Autodesk Inventor part; units mm, degrees
ref_plane "Work Plane1" through (1.7107, 0, 1.8263) normal (1, 0, 0) x (0, 0, -1)
ref_plane "YZ Plane" through (0, 0, 0) normal (1, 0, 0) x (0, 1, 0)
ref_plane "XZ Plane" through (0, 0, 0) normal (0, 1, 0) x (-1, 0, 0)
sketch "Sketch1" plane through (0, 0, 0) normal (0, 1, 0) x (-1, 0, 0)
  line L0 (0, 0) -> (2.6987, 0) construction
  line L1 (2.6987, 0) -> (2.6987, -2.7407) construction
  line L2 (2.6987, -2.7407) -> (0, -2.7407) construction
  line L3 (0, -2.7407) -> (0, 0) construction
  line L4 (2.6987, 0) -> (2.6987, -1.8263) construction
  line L5 (2.6987, 0) -> (4.525, 0) construction
  arc A0 (0, -2.7407) -> (2.6987, -1.8263) centre (0, 1.6991) ccw
  line L6 (2.6987, -1.8263) -> (2.6987, 0)
  arc A1 (-2.6987, -1.8263) -> (0, -2.7407) centre (0, 1.6991) ccw
  line L7 (-2.6987, -1.8263) -> (-2.6987, 0)
  arc A2 (2.6987, 1.8263) -> (0, 2.7407) centre (0, -1.6991) ccw
  line L8 (2.6987, 1.8263) -> (2.6987, 0)
  arc A3 (0, 2.7407) -> (-2.6987, 1.8263) centre (0, -1.6991) ccw
  line L9 (-2.6987, 1.8263) -> (-2.6987, 0)
  dimension "d0" = 2.6987
  dimension "d1" = 2.7407
  dimension "d2" = 1.8263
  dimension "d3" = 90
extrude "Extrusion1" add sketch "Sketch1" along normal blind 7.8334
sketch "Sketch2" plane through (0, 0, 0) normal (0, -1, 0) x (1, 0, 0)
  circle A0 centre (0, 0) radius 1.5862
  dimension "d6" = 3.1725
extrude "Extrusion2" cut sketch "Sketch2" against normal blind 4.0589
ref_plane "Work Plane1" through (1.7107, 0, 1.8263) normal (1, 0, 0) x (0, 0, -1)
sketch "Sketch3" plane through (1.7107, 0, 1.8263) normal (1, 0, 0) x (0, 0, -1)
  line L0 (3.6525, 7.8334) -> (0, 7.8334)
  line L1 (3.6525, 7.8334) -> (0, 7.8334)
  line L2 (0, 7.8334) -> (0, 9.3066)
  line L3 (0, 9.3066) -> (1.8263, 9.3066) construction
  line L4 (3.6525, 9.3066) -> (3.6525, 7.8334)
  arc A0 (0.7459, 12.8145) -> (2.9066, 12.8145) centre (1.8263, 11.7342) ccw
  line L5 (1.8263, 11.7342) -> (1.8263, 14.772) construction
  line L6 (2.9066, 12.8145) -> (3.9743, 13.8822)
  line L7 (0.7459, 12.8145) -> (-0.3218, 13.8822)
  arc A1 (-0.3218, 13.8822) -> (0, 9.3066) centre (1.8263, 11.7342) ccw
  arc A2 (3.6525, 9.3066) -> (3.9743, 13.8822) centre (1.8263, 11.7342) ccw
  point P0 (1.8263, 0)
  dimension "d10" = 1.4732
  dimension "d12" = 3.0556
  dimension "d13" = 45
  dimension "d14" = 45
extrude "Extrusion3" add sketch "Sketch3" against normal blind 3.2385
properties part number "hand project" material "ABS Plastic"
The model under review builds one solid part; all positions refer to its coordinate system, in mm. A direction names the side the tool comes from. Give positions to 0.01 mm unless a question says otherwise; leave off trailing zeros. Write each loop counter-clockwise with the first axis right and the second up, starting at its lowest first coordinate (ties: lowest second). Pieces come first, ordered by that corner, then holes.
(1) Consider section A-A, the plane y = 2.75. Give the boundary of the cut face in (x, z).
(2) For P1, Ø1.2, axis at x = -0.5, y = 8.5, coming from the +Z side; P2, Ø2.5, axis at x = 0.5, z = 0.5, coming from the +Y side; P3, Ø0.7, axis at x = 0.5, y = 8.5, coming from the -Z side; P4, Ø3, axis at x = 2, z = 1.5, coming from the -Y side, all flat-tipped, find the tip position at first contact; note any pin that passes through.
(3) To check wall thickness, follow L1, parallel to Z at x = 0, y = 1.25; L2, parallel to Y at x = -2.1, z = 0; L3, parallel to X at y = 10.5, z = -1.75. State the ranges of each line that lie inside material, in increasing order.
(4) The part is to be moulded in two halves that separate along Z. For faces 5 (the cylindrical face through (0.114, 10.207, 0.05)), 6 (the flat face through (0, 9, 1.826)), 7 (the flat face through (-1.528, 10, -1)), say which applies: released by +Z, released by -Z, zero draft, split by the parting line, or undercut.
(5) Consider section B-B, the plane z = -2.5. Give the boundary of the cut face in (x, y), and give its area (3 significant figures).
(6) Tool access review of faces 1 (the cylindrical face through (-1.44, 3.86, -2.5)), 2 (the cylindrical face through (1.41, 3.86, -2.51)), 3 (the flat face through (0, 9, -1.826)), 4 (the cylindrical face through (-0.34, 2, -1.55)): name each direction out of +Z, -Z, +X, -X, +Y, -Y from which nothing blocks a thin tool from reaching the whole face with its end or side.
(7) Consider section D-D, the plane z = 0. Give the boundary of the cut face in (x, y), and give its area (3 significant figures).
(8) Consider section C-C, the plane y = 11.5. Give the boundary of the cut face in (x, z), and give its area (3 significant figures).
Returned:
1. outline: (-2.7, -1.83) arc R4.44 ccw to (0, -2.74) arc R4.44 ccw to (2.7, -1.83) - (2.7, 1.83) arc R4.44 ccw to (0, 2.74) arc R4.44 ccw to (-2.7, 1.83) - close; hole circle Ø3.17 at (0, 0)
2. P1: stops at z = 1.83
2. P2: stops at y = 13.48
2. P3: stops at z = -1.83
2. P4: stops at y = 0
3. L1: z = -2.74 to -1.59, 1.59 to 2.74
3. L2: y = 0 to 7.83
3. L3: x = -1.53 to 1.71
4. face 5: undercut
4. face 6: released by +Z
4. face 7: zero draft
5. outline: (-1.53, 10.01) - (1.71, 10.01) - (1.71, 13.46) - (-1.53, 13.46) - close; (-1.44, 0) - (1.44, 0) - (1.44, 7.83) - (-1.44, 7.83) - close
5. area: 33.8 mm2
6. face 1: -Z, -X, -Y
6. face 2: -Z, +X, -Y
6. face 3: -Z, +X, -X
6. face 4: -Y
7. outline: (-2.7, 0) - (-1.59, 0) - (-1.59, 4.06) - (1.59, 4.06) - (1.59, 0) - (2.7, 0) - (2.7, 7.83) - (1.71, 7.83) - (1.71, 10.21) - (-1.53, 10.21) - (-1.53, 7.83) - (-2.7, 7.83) - close
7. area: 37.1 mm2
8. outline: (-1.53, -3.03) - (1.71, -3.03) - (1.71, -1.51) - (-1.53, -1.51) - close; (-1.53, 1.51) - (1.71, 1.51) - (1.71, 3.03) - (-1.53, 3.03) - close
8. area: 9.84 mm2
